```python
from build123d import *

# Parameters (mm, degrees)
SKETCH_1_W                  = 80
SKETCH_1_H                  = 65
EXTRUDE_1_DEPTH             = 3
SKETCH_2_R                  = 2.1
CUT_EXTRUDE_1_DEPTH         = 52.626059311
PATTERN_LINEAR_1_COUNT      = 2
PATTERN_LINEAR_1_PITCH      = 20
PATTERN_LINEAR_1_COUNT_DIR2 = 2
PATTERN_LINEAR_1_PITCH_DIR2 = 35
SKETCH_4_W                  = 20.5
SKETCH_4_H                  = 40.5
CUT_EXTRUDE_2_DEPTH         = 3
FILLET_1_R                  = 1
CUT_EXTRUDE_3_REACH         = 53.626
SKETCH_5_R                  = 2.1
CHAMFER_3_SIZE              = 5


with BuildPart() as part:
    # 草圖1 → 填料-伸長1 (new body)
    with BuildSketch(Plane.XY):
        Rectangle(SKETCH_1_W, SKETCH_1_H)
    extrude(amount=EXTRUDE_1_DEPTH)

    # 草圖2 → 除料-伸長1 (cut, through all)
    with BuildSketch(Plane.XY.offset(3)):
        with Locations((-30, 17.5)):
            Circle(SKETCH_2_R)
    cut_extrude_1 = extrude(amount=-CUT_EXTRUDE_1_DEPTH, mode=Mode.SUBTRACT)

    # 直線複製排列1: Cut-Extrude 1 2 × 2
    with Locations(*[(i * PATTERN_LINEAR_1_PITCH, -j * PATTERN_LINEAR_1_PITCH_DIR2, 0) for i in range(PATTERN_LINEAR_1_COUNT) for j in range(PATTERN_LINEAR_1_COUNT_DIR2) if (i, j) != (0, 0)]):
        add(cut_extrude_1, mode=Mode.SUBTRACT)

    # 草圖4 → 除料-伸長2 (cut)
    with BuildSketch(Plane.XY.offset(3)):
        with Locations((22.75, 0)):
            Rectangle(SKETCH_4_W, SKETCH_4_H)
    extrude(amount=-CUT_EXTRUDE_2_DEPTH, mode=Mode.SUBTRACT)

    # 圓角1
    fillet_1_edges = [part.edges().sort_by_distance(p)[0] for p in [
        (33, 20.25, 1.5),
        (33, -20.25, 1.5),
        (12.5, -20.25, 1.5),
        (12.5, 20.25, 1.5),
    ]]
    fillet(fillet_1_edges, radius=FILLET_1_R)

    # 草圖5 → 除料-伸長3 (cut, up to next)
    with BuildSketch(Plane.XY.offset(3), mode=Mode.PRIVATE) as cut_extrude_3_sk1:
        with Locations((17.75, 24.9)):
            Circle(SKETCH_5_R)
    cut_extrude_3_tool1 = extrude(cut_extrude_3_sk1.sketch, amount=-CUT_EXTRUDE_3_REACH, mode=Mode.PRIVATE) & part.part
    # 草圖5 → 除料-伸長3 (cut, up to next)
    with BuildSketch(Plane.XY.offset(3), mode=Mode.PRIVATE) as cut_extrude_3_sk2:
        with Locations((27.75, 24.9)):
            Circle(SKETCH_5_R)
    cut_extrude_3_tool2 = extrude(cut_extrude_3_sk2.sketch, amount=-CUT_EXTRUDE_3_REACH, mode=Mode.PRIVATE) & part.part
    # 草圖5 → 除料-伸長3 (cut, up to next)
    with BuildSketch(Plane.XY.offset(3), mode=Mode.PRIVATE) as cut_extrude_3_sk3:
        with Locations((27.75, -24.6)):
            Circle(SKETCH_5_R)
    cut_extrude_3_tool3 = extrude(cut_extrude_3_sk3.sketch, amount=-CUT_EXTRUDE_3_REACH, mode=Mode.PRIVATE) & part.part
    # 草圖5 → 除料-伸長3 (cut, up to next)
    with BuildSketch(Plane.XY.offset(3), mode=Mode.PRIVATE) as cut_extrude_3_sk4:
        with Locations((17.75, -24.6)):
            Circle(SKETCH_5_R)
    cut_extrude_3_tool4 = extrude(cut_extrude_3_sk4.sketch, amount=-CUT_EXTRUDE_3_REACH, mode=Mode.PRIVATE) & part.part
    add(cut_extrude_3_tool1.solids().sort_by_distance((17.75, 24.9, 3))[0], mode=Mode.SUBTRACT)
    add(cut_extrude_3_tool2.solids().sort_by_distance((27.75, 24.9, 3))[0], mode=Mode.SUBTRACT)
    add(cut_extrude_3_tool3.solids().sort_by_distance((27.75, -24.6, 3))[0], mode=Mode.SUBTRACT)
    add(cut_extrude_3_tool4.solids().sort_by_distance((17.75, -24.6, 3))[0], mode=Mode.SUBTRACT)

    # 導角3
    chamfer_3_edges = [part.edges().sort_by_distance(p)[0] for p in [
        (-40, 32.5, 1.5),
        (40, 32.5, 1.5),
        (40, -32.5, 1.5),
        (-40, -32.5, 1.5),
    ]]
    chamfer(chamfer_3_edges, length=CHAMFER_3_SIZE)


solid = part.part
```
Input: part model. Units: mm. Frame: model coordinates. A direction names the side the tool comes from. Give positions to 0.01 mm unless a question says otherwise; leave off trailing zeros. Order: outer loops, then holes, each group sorted by start corner. A loop starts at its lowest first (then second) coordinate and runs counter-clockwise, first axis right, second up. Notation, with made-up numbers: M 63,50.25 L 106,50.25 A19 ccw 106,65.25 Z; hole C -19.75,50.25 d8. An arc over 180 degrees is marked long. One line per question, with ' | ' between items. Start each with the question number.
1. First-contact query: pin 1 Ø5 at (x, y) = (-30, 17.5) entering from -Z. Flat tip, straight axial feed; report the tip coordinate or a pass-through.
2. Material intervals for probe 1 along Y at (x, z) = (27.75, 1.7); probe 2 along X at (y, z) = (6, 2.65); probe 3 along Y at (x, z) = (14, 1.35), sorted ascending. Write a range as [from, to].
3. Pull-direction query (X, two-part tool) for faces 1 (the face through (37.5, 30, 1.5)), 2 (the face through (18.88, -22.83, 1.52)), 3 (the face through (-1, 0, 0)); classes: released by +X, released by -X, zero draft, split by the parting line, or undercut.
4. Section query A-A (y = 4.5). Return the cut outline in (x, z).
5. Access query for faces 4 (the face through (-37.5, 30, 1.5)), 5 (the face through (12.5, 0, 2)). Directions: +Z, -Z, +X, -X, +Y, -Y. A direction counts if a zero-diameter tool reaches every point of the face in a straight line with its end or side. Return the directions, or none.
6. Section query D-D (x = -30). Return the cut outline in (y, z).
7. Section query C-C (y = 17.5). Return the cut outline in (x, z), and give its area (3 significant figures).
8. Section query B-B (x = 24.5). Return the cut outline in (y, z).
Here are the results:
1) pin 1: z = 0
2) probe 1: [-32.5, -26.7], [-22.5, -20.25], [20.25, 22.8], [27, 32.5] | probe 2: [-40, 12.5], [33, 40] | probe 3: [-32.5, -20.25], [20.25, 32.5]
3) face 1: released by +X | face 2: undercut | face 3: zero draft
4) outline: M -40,0 L 12.5,0 L 12.5,3 L -40,3 Z; M 33,0 L 40,0 L 40,3 L 33,3 Z
5) face 4: +Z, -Z, -X, +Y | face 5: +Z, -Z
6) outline: M -32.5,0 L -19.6,0 L -19.6,3 L -32.5,3 Z; M -15.4,0 L 15.4,0 L 15.4,3 L -15.4,3 Z; M 19.6,0 L 32.5,0 L 32.5,3 L 19.6,3 Z
7) outline: M -40,0 L -32.1,0 L -32.1,3 L -40,3 Z; M -27.9,0 L -12.1,0 L -12.1,3 L -27.9,3 Z; M -7.9,0 L 12.5,0 L 12.5,3 L -7.9,3 Z; M 33,0 L 40,0 L 40,3 L 33,3 Z | area: 153 mm²
8) outline: M -32.5,0 L -20.25,0 L -20.25,3 L -32.5,3 Z; M 20.25,0 L 32.5,0 L 32.5,3 L 20.25,3 Z
